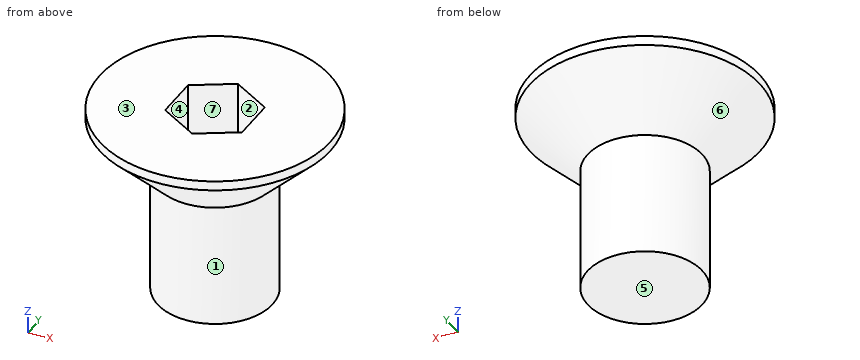
Autodesk Inventor part; units mm, degrees
ref_plane "YZ Plane" through (0, 0, 0) normal (1, 0, 0) x (0, 1, 0)
ref_plane "XZ Plane" through (0, 0, 0) normal (0, 1, 0) x (-1, 0, 0)
ref_plane "XY Plane" through (0, 0, 0) normal (0, 0, 1) x (1, 0, 0)
sketch "スケッチ1" plane through (0, 0, 0) normal (0, 0, 1) x (1, 0, 0)
  circle A0 centre (0, 0) radius 1.5
  dimension "d0" = 3
extrude "押し出し1" add sketch "スケッチ1" along normal blind 5
thread "ねじ1"
sketch "スケッチ2" plane through (0, 0, 5) normal (0, 0, 1) x (1, 0, 0)
  circle A0 centre (0, 0) radius 3
  dimension "d5" = 6
extrude "押し出し2" add sketch "スケッチ2" against normal blind 1.75
chamfer "面取り1" distance 1.5 angle 45 1 edges at (-3, 0, 3.25)
sketch "スケッチ3" plane through (0, 0, 5) normal (0, 0, 1) x (1, 0, 0)
  line L0 (0, 1.1547) -> (1, 0.5774)
  line L1 (1, 0.5774) -> (1, -0.5774)
  line L2 (1, -0.5774) -> (0, -1.1547)
  line L3 (0, -1.1547) -> (-1, -0.5774)
  line L4 (-1, -0.5774) -> (-1, 0.5774)
  line L5 (-1, 0.5774) -> (0, 1.1547)
  point P0 (0, 0)
  point P1 (0, 0)
  dimension "d11" = 2
extrude "押し出し3" cut sketch "スケッチ3" against normal blind 1.5
properties part number "m3皿ネジ5 (1)" material "鉄 灰色"
Geometry check sheet. Reference: the model listing, model coordinates, mm. Face numbers are marked on the shaded views. A direction names the side the tool comes from. Round coordinates to 2 decimals unless told otherwise and drop trailing zeros. Order: outer loops, then holes, each group sorted by start corner. A loop starts at its lowest first (then second) coordinate and runs counter-clockwise, first axis right, second up. Notation, with made-up numbers: (54.5, 0.5) -> (112.5, 0.5) arc R22 cw to (112.5, 11.5) -> close; hole circle Ø11 at (-13, 0.25). An arc over 180 degrees is marked (long way). Return JSON: item names as keys, results as strings. Group by question number.
Q1. Section check D-D, the plane z = 4.5. Record the boundary of the cut face in (x, y).
Q2. Material ranges on probe 1 along Y at (x, z) = (0.5, 3.9); probe 2 along Z at (x, y) = (-1.75, 0); probe 3 along Y at (x, z) = (0.6, 4.25), recorded low to high. Write a range as from..to.
Q3. Tool access check on the marked faces 1, 2 and 3. Record the directions out of +Z, -Z, +X, -X, +Y, -Y that give a thin tool (end or side, any length) a straight path to the whole face; none if there is none.
Q4. Release check for a two-part mould opening along Y. For the marked faces 4, 5, 6 and 7 record: released by +Y, released by -Y, zero draft, split by the parting line, or undercut.
Q5. Section check B-B, the plane z = 4. Record the boundary of the cut face in (x, y).
Q6. Gauge pin test, flat end, axial feed: pin 1 (1 mm diameter, centred on y = -2, z = 4.5, fed in from -X). Record the tip position at first contact, or that the pin passes through.
Q7. Section check C-C, the plane z = 0.8. Record the boundary of the cut face in (x, y), plus the area to 3 significant figures.
Numbers:
{
 "1": {"outline": "circle Ø5.5 at (0, 0); hole (-1, -0.58) -> (0, -1.15) -> (1, -0.58) -> (1, 0.58) -> (0, 1.15) -> (-1, 0.58) -> close"},
 "2": {"probe 1": "-2.09..-0.87, 0.87..2.09", "probe 2": "3.5..5", "probe 3": "-2.43..-0.81, 0.81..2.43"},
 "3": {"face 1": "-Z", "face 2": "+Z", "face 3": "+Z, +X, -X, +Y, -Y"},
 "4": {"face 4": "undercut", "face 5": "zero draft", "face 6": "split by the parting line", "face 7": "undercut"},
 "5": {"outline": "circle Ø4.5 at (0, 0); hole (-1, -0.58) -> (0, -1.15) -> (1, -0.58) -> (1, 0.58) -> (0, 1.15) -> (-1, 0.58) -> close"},
 "6": {"pin 1": "x = -2.56"},
 "7": {"outline": "circle Ø3 at (0, 0)", "area": "7.07 mm^2"}
}
